Design review of the part built by this model. Coordinates are the model's own, in mm. A direction names the side the tool comes from. Give positions to 0.01 mm unless a question says otherwise; leave off trailing zeros. Loops run counter-clockwise (first coordinate to the right, second up) from the corner with the lowest first, then second, coordinate; pieces in that order, holes last. Notation, with made-up numbers: (2, 88) -> (23, 88) arc R27 cw to (23, 116) -> close; hole circle Ø9 at (56, 29.5). An arc over 180 degrees is marked (long way). Use a Markdown table: item, result. Add a question column.
1. Add section B-B (x = -31). State the section outline as (y, z) points (3 decimals).
2. For pin 1 Ø1.2 at (x, y) = (26, -1.5) entering from +Z (3 decimals); pin 2 Ø2 at (y, z) = (11, 46) entering from +X; pin 3 Ø9 at (x, z) = (-21, 95) entering from +Y; pin 4 Ø0.8 at (y, z) = (11, -7.5) entering from -X, all flat-tipped, find the tip position at first contact; note any pin that passes through.
3. Draft analysis for pull direction Z (two halves, no side actions). For faces 5 (the cylindrical face through (64.1, 0.71, -91.33)), 6 (the flat face through (-77, 0, -9)), 7 (the cylindrical face through (67.18, -1.23, 101.39)), 8 (the cylindrical face through (76.96, 4.73, -120.45)), state which applies: pulls with the +Z half, pulls with the -Z half, needs draft (parallel to the pull), parting line crosses it, or undercut.
4. Add section A-A (z = 68). State the section outline as (x, y) points.
5. Add section C-C (y = 4.75). State the section outline as (x, z) points (3 decimals), and give its area (3 significant figures).
6. For faces 1 (the cylindrical face through (64.29, 0.71, 98.55)), 2 (the cylindrical face through (66.93, -1.23, -94.23)), 3 (the cylindrical face through (-67.18, -1.23, -93.98)), 4 (the flat face through (1, 1.4, -103)), list the 3-axis set-ups (+Z, -Z, +X, -X, +Y, -Y) from which the entire face can be reached by the end or side of a thin tool; tool diameter is ignored.
7. To check wall thickness, follow line 1 (Z direction, x = 30.5, y = 5) (3 decimals); line 2 (Z direction, x = -45.5, y = 0.75) (3 decimals); line 3 (X direction, y = 4.25, z = 47). State the ranges of each line that lie inside material, in increasing order.
```python
from build123d import *

# Parameters (mm, degrees)
F1_DEPTH  = 9.6
F3_DEPTH  = 10
F5_DEPTH  = 2.5
F6_DEPTH  = 68.834
F7_SIZE   = 2.5
F9_DEPTH  = 8.2
F11_DEPTH = 2.5


with BuildPart() as f1:
    # F0 (on Front) → F1 (new body)
    with BuildSketch(Plane.XZ):
        with BuildLine():
            Line((71.63, 122.625), (-71.63, 122.625))
            ThreePointArc((-71.63, 122.625), (-77.018154, 120.393154), (-79.25, 115.005))
            Line((-79.25, 115.005), (-79.25, -115.005))
            ThreePointArc((-79.25, -115.005), (-77.018154, -120.393154), (-71.63, -122.625))
            Line((-71.63, -122.625), (71.63, -122.625))
            ThreePointArc((71.63, -122.625), (77.018154, -120.393154), (79.25, -115.005))
            Line((79.25, -115.005), (79.25, 115.005))
            ThreePointArc((79.25, 115.005), (77.018154, 120.393154), (71.63, 122.625))
        make_face()
    extrude(amount=-F1_DEPTH)

    # F2 (on face) → F3 (cut)
    with BuildSketch(Plane.XZ):
        with BuildLine():
            Line((55.6088, 102.205), (-55.6088, 102.205))
            ThreePointArc((-55.6088, 102.205), (-64.193925, 98.648925), (-67.75, 90.0638))
            Line((-67.75, 90.0638), (-67.75, -82.6538))
            ThreePointArc((-67.75, -82.6538), (-64.193925, -91.238925), (-55.6088, -94.795))
            Line((-55.6088, -94.795), (55.6088, -94.795))
            ThreePointArc((55.6088, -94.795), (64.193925, -91.238925), (67.75, -82.6538))
            Line((67.75, -82.6538), (67.75, 90.0638))
            ThreePointArc((67.75, 90.0638), (64.193925, 98.648925), (55.6088, 102.205))
        make_face()
    extrude(amount=-F3_DEPTH, mode=Mode.SUBTRACT)

    # F4 (on face) → F5 (join)
    with BuildSketch(Plane.XZ):
        with BuildLine():
            Line((55.6088, 106.255), (-55.6088, 106.255))
            ThreePointArc((-55.6088, 106.255), (-67.057707, 101.512707), (-71.8, 90.0638))
            Line((-71.8, 90.0638), (-71.8, -82.6538))
            ThreePointArc((-71.8, -82.6538), (-67.057707, -94.102707), (-55.6088, -98.845))
            Line((-55.6088, -98.845), (55.6088, -98.845))
            ThreePointArc((55.6088, -98.845), (67.057707, -94.102707), (71.8, -82.6538))
            Line((71.8, -82.6538), (71.8, 90.0638))
            ThreePointArc((71.8, 90.0638), (67.057707, 101.512707), (55.6088, 106.255))
        make_face()
    extrude(amount=F5_DEPTH)

    # F2 (on face) → F6 (cut)
    with BuildSketch(Plane.XZ):
        with BuildLine():
            Line((55.6088, 102.205), (-55.6088, 102.205))
            ThreePointArc((-55.6088, 102.205), (-64.193925, 98.648925), (-67.75, 90.0638))
            Line((-67.75, 90.0638), (-67.75, -82.6538))
            ThreePointArc((-67.75, -82.6538), (-64.193925, -91.238925), (-55.6088, -94.795))
            Line((-55.6088, -94.795), (55.6088, -94.795))
            ThreePointArc((55.6088, -94.795), (64.193925, -91.238925), (67.75, -82.6538))
            Line((67.75, -82.6538), (67.75, 90.0638))
            ThreePointArc((67.75, 90.0638), (64.193925, 98.648925), (55.6088, 102.205))
        make_face()
    extrude(amount=F6_DEPTH, mode=Mode.SUBTRACT)

    # F7
    f7_edges = [f1.edges().sort_by_distance(p)[0] for p in [
        (67.75, -2.5, 3.705),
    ]]
    chamfer(f7_edges, length=F7_SIZE)

    # F8 (on face) → F9 (cut)
    with BuildSketch(Plane(origin=(0, 9.6, 0), x_dir=(-1, 0, 0), z_dir=(0, 1, 0))):
        with BuildLine():
            Line((65.75, 107.625), (-65.75, 107.625))
            ThreePointArc((-65.75, 107.625), (-67.164214, 107.039214), (-67.75, 105.625))
            Line((-67.75, 105.625), (-67.75, -109.375))
            ThreePointArc((-67.75, -109.375), (-67.164214, -110.789214), (-65.75, -111.375))
            Line((-65.75, -111.375), (65.75, -111.375))
            ThreePointArc((65.75, -111.375), (67.164214, -110.789214), (67.75, -109.375))
            Line((67.75, -109.375), (67.75, 105.625))
            ThreePointArc((67.75, 105.625), (67.164214, 107.039214), (65.75, 107.625))
        make_face()
    extrude(amount=-F9_DEPTH, mode=Mode.SUBTRACT)

    # F10 (on face) → F11 (join)
    with BuildSketch(Plane(origin=(0, 9.6, 0), x_dir=(-1, 0, 0), z_dir=(0, 1, 0))):
        with BuildLine():
            Line((73.05, 94.875), (73, 94.875))
            ThreePointArc((73, 94.875), (71.585786, 94.289214), (71, 92.875))
            Line((71, 92.875), (71, -76.125))
            ThreePointArc((71, -76.125), (71.585786, -77.539214), (73, -78.125))
            Line((73, -78.125), (73.05, -78.125))
            ThreePointArc((73.05, -78.125), (74.464214, -77.539214), (75.05, -76.125))
            Line((75.05, -76.125), (75.05, 92.875))
            ThreePointArc((75.05, 92.875), (74.464214, 94.289214), (73.05, 94.875))
        make_face()
    extrude(amount=F11_DEPTH)


solid = f1.part
```
Taken from the geometry:
| question | item | result |
|---|---|---|
| 1 | outline | (-2.5, -98.845) -> (0, -98.845) -> (0, -122.625) -> (9.6, -122.625) -> (9.6, -111.375) -> (1.4, -111.375) -> (1.4, -94.795) -> (0, -94.795) -> (-2.5, -97.295) -> close; (-2.5, 104.705) -> (0, 102.205) -> (1.4, 102.205) -> (1.4, 107.625) -> (9.6, 107.625) -> (9.6, 122.625) -> (0, 122.625) -> (0, 106.255) -> (-2.5, 106.255) -> close |
| 2 | pin 1 | stops at z = 106.255 |
| 2 | pin 2 | stops at x = -71 |
| 2 | pin 3 | passes through |
| 2 | pin 4 | stops at x = -75.05 |
| 3 | face 5 | undercut |
| 3 | face 6 | needs draft |
| 3 | face 7 | pulls with the +Z half |
| 3 | face 8 | pulls with the -Z half |
| 4 | outline | (-79.25, 0) -> (-71.8, 0) -> (-71.8, -2.5) -> (-70.25, -2.5) -> (-67.75, 0) -> (-67.75, 9.6) -> (-71, 9.6) -> (-71, 12.1) -> (-75.05, 12.1) -> (-75.05, 9.6) -> (-79.25, 9.6) -> close; (67.75, 0) -> (70.25, -2.5) -> (71.8, -2.5) -> (71.8, 0) -> (79.25, 0) -> (79.25, 9.6) -> (67.75, 9.6) -> close |
| 5 | outline | (-79.25, -115.005) arc R7.62 ccw to (-71.63, -122.625) -> (71.63, -122.625) arc R7.62 ccw to (79.25, -115.005) -> (79.25, 115.005) arc R7.62 ccw to (71.63, 122.625) -> (-71.63, 122.625) arc R7.62 ccw to (-79.25, 115.005) -> close; hole (-67.75, -109.375) arc R2 ccw to (-65.75, -111.375) -> (65.75, -111.375) arc R2 ccw to (67.75, -109.375) -> (67.75, 105.625) arc R2 ccw to (65.75, 107.625) -> (-65.75, 107.625) arc R2 ccw to (-67.75, 105.625) -> close |
| 5 | area | 9,150 mm^2 |
| 6 | face 1 | +Y, -Y |
| 6 | face 2 | -Z, +X, -Y |
| 6 | face 3 | -Z, -X, -Y |
| 6 | face 4 | +Y |
| 7 | line 1 | z = -122.625 to -111.375, 107.625 to 122.625 |
| 7 | line 2 | z = -122.625 to -94.795, 102.205 to 122.625 |
| 7 | line 3 | x = -79.25 to -67.75, 67.75 to 79.25 |
